```python
from build123d import *

# Parameters (mm, degrees)
SKETCH1_W           = 7.62
SKETCH1_H           = 12.7
BOSS_EXTRUDE1_DEPTH = 457.2
SKETCH3_R           = 1.905
CUT_EXTRUDE2_DEPTH  = 15
SKETCH4_W           = 16.186958623
SKETCH4_H           = 8.82047947
CUT_EXTRUDE3_DEPTH  = 15
CUT_EXTRUDE4_DEPTH  = 15
FILLET1_R           = 2.5
SKETCH6_W           = 7.62
SKETCH6_H           = 12.7
BOSS_EXTRUDE2_DEPTH = 80
SKETCH7_W           = 12.13309825
SKETCH7_H           = 9.938189712
CUT_EXTRUDE5_DEPTH  = 80
CUT_EXTRUDE6_DEPTH  = 80
FILLET2_R           = 2.5


with BuildPart() as part:
    # Sketch1 → Boss-Extrude1 (new body)
    with BuildSketch(Plane.XY):
        with Locations((3.81, 6.35)):
            Rectangle(SKETCH1_W, SKETCH1_H)
    extrude(amount=BOSS_EXTRUDE1_DEPTH)

    # Sketch3 → Cut-Extrude2 (cut)
    with BuildSketch(Plane(origin=(7.62, 0, 0), x_dir=(0, 0, -1), z_dir=(1, 0, 0))):
        with Locations((-228.6, 6.35)):
            Circle(SKETCH3_R)
    extrude(amount=-CUT_EXTRUDE2_DEPTH, mode=Mode.SUBTRACT)

    # Sketch4 → Cut-Extrude3 (cut)
    with BuildSketch(Plane(origin=(7.62, 0, 0), x_dir=(0, 0, -1), z_dir=(1, 0, 0))):
        with Locations((-449.106520689, 6.226228187)):
            Rectangle(SKETCH4_W, SKETCH4_H)
    extrude(amount=-CUT_EXTRUDE3_DEPTH, mode=Mode.SUBTRACT)

    # Sketch5 → Cut-Extrude4 (cut)
    with BuildSketch(Plane(origin=(0, 12.7, 0), x_dir=(1, 0, 0), z_dir=(0, 1, 0))):
        with BuildLine():
            ThreePointArc((5.157644125, -452.042355875), (2.462355875, -452.042355875), (2.462355875, -454.737644125))
            Line((2.462355875, -454.737644125), (5.157644125, -452.042355875))
        make_face()
        with BuildLine():
            Line((5.157644125, -452.042355875), (2.462355875, -454.737644125))
            ThreePointArc((2.462355875, -454.737644125), (4.539339745, -455.150781904), (5.715856599, -453.39))
            ThreePointArc((5.715856599, -453.39), (5.570781904, -452.660660255), (5.157644125, -452.042355875))
        make_face()
    extrude(amount=-CUT_EXTRUDE4_DEPTH, mode=Mode.SUBTRACT)

    # Fillet1
    fillet1_edges = [part.edges().sort_by_distance(p)[0] for p in [
        (7.62, 0.907994226, 457.2),
        (0, 0.907994226, 457.2),
        (7.62, 11.668233961, 457.2),
        (0, 11.668233961, 457.2),
    ]]
    fillet(fillet1_edges, radius=FILLET1_R)

    # Sketch6 → Boss-Extrude2 (add)
    with BuildSketch(Plane(origin=(0, 0, 0), x_dir=(-1, 0, 0), z_dir=(0, 0, -1))):
        with Locations((-3.81, 6.35)):
            Rectangle(SKETCH6_W, SKETCH6_H)
    extrude(amount=BOSS_EXTRUDE2_DEPTH)

    # Sketch7 → Cut-Extrude5 (cut)
    with BuildSketch(Plane(origin=(7.62, 0, 0), x_dir=(0, 0, -1), z_dir=(1, 0, 0))):
        with Locations((73.933450875, 6.395782886)):
            Rectangle(SKETCH7_W, SKETCH7_H)
    extrude(amount=-CUT_EXTRUDE5_DEPTH, mode=Mode.SUBTRACT)

    # Sketch8 → Cut-Extrude6 (cut)
    with BuildSketch(Plane(origin=(0, 12.7, 0), x_dir=(1, 0, 0), z_dir=(0, 1, 0))):
        with BuildLine():
            ThreePointArc((5.796561175, 76.108438825), (4.620573114, 77.868429334), (2.544522757, 77.455477243))
            Line((2.544522757, 77.455477243), (5.238599594, 74.761400406))
            ThreePointArc((5.238599594, 74.761400406), (5.651551685, 75.379426886), (5.796561175, 76.108438825))
        make_face()
        with BuildLine():
            Line((5.238599594, 74.761400406), (2.544522757, 77.455477243))
            ThreePointArc((2.544522757, 77.455477243), (2.544522757, 74.761400406), (5.238599594, 74.761400406))
        make_face()
    extrude(amount=-CUT_EXTRUDE6_DEPTH, mode=Mode.SUBTRACT)

    # Fillet2
    fillet2_edges = [part.edges().sort_by_distance(p)[0] for p in [
        (0, 0.713344015, -80),
        (7.62, 12.032438871, -80),
        (0, 12.032438871, -80),
        (7.62, 0.713344015, -80),
    ]]
    fillet(fillet2_edges, radius=FILLET2_R)


solid = part.part
```
The listing builds one solid part. Answer for the finished solid, in the listing's coordinates (mm). Coordinates: 2 decimals unless noted, no trailing zeros. Return JSON: item names as keys, results as strings. Group by question number.
(1) A cutting plane is placed at A-A on x = 3.81. Count the separate pieces of the cut face and the enclosed holes in it, and give its area (3 significant figures).
(2) Find the intervals of material crossed by probe 1 along Z at (x, y) = (3.5, 1.5); probe 2 along Y at (x, z) = (2, 228.6) (3 decimals); probe 3 along Z at (x, y) = (6.25, 2.5), in increasing order. Write a range as from..to.
(3) Given pin 1 Ø2.5 at (x, y) = (5.5, 4.5) entering from +Z, flat-ended and moving along its own axis, determine where the tip first touches the part or whether it passes through.
The answers:
{
 "1": {"separate pieces": "5", "enclosed holes": "1", "area": "6,520 mm^2"},
 "2": {"probe 1": "z = -67.87..451.51, 455.27..457.2", "probe 2": "y = 0..4.445, 8.255..12.7", "probe 3": "z = -67.87..441.01"},
 "3": {"pin 1": "stops at z = 441.01"}
}
